Autodesk Inventor part; units mm, degrees
ref_plane "YZ Plane" through (0, 0, 0) normal (1, 0, 0) x (0, 1, 0)
ref_plane "XZ Plane" through (0, 0, 0) normal (0, 1, 0) x (-1, 0, 0)
ref_plane "XY Plane" through (0, 0, 0) normal (0, 0, 1) x (1, 0, 0)
sketch "Sketch1" plane through (0, 0, 0) normal (0, 0, 1) x (1, 0, 0)
  circle A0 centre (0, 0) radius 18.5
  dimension "d0" = 37
extrude "Extrusion1" add sketch "Sketch1" along normal blind 85
sketch "Sketch2" plane through (0, 0, 85) normal (0, 0, 1) x (1, 0, 0)
  circle A0 centre (0, -7) radius 3
  point P0 (0, 0)
  dimension "d3" = 6
  dimension "d4" = 7
extrude "Extrusion2" add sketch "Sketch2" along normal blind 21
sketch "Sketch3" plane through (0, 0, 85) normal (0, 0, 1) x (1, 0, 0)
  circle A0 centre (0, -7) radius 3
  circle A1 centre (0, -7) radius 6
  point P0 (0, 0)
  dimension "d7" = 12
extrude "Extrusion3" add sketch "Sketch3" along normal blind 6
sketch "Sketch4" plane through (0, -7, 106) normal (0, 0, 1) x (1, 0, 0)
  circle A0 centre (0, 0) radius 3
  line L0 (-1.8, 2.4) -> (1.8, 2.4)
  point P0 (0, 7)
  dimension "d10" = 2.4
extrude "Extrusion4" cut sketch "Sketch4" against normal blind 12 contours L0 A0 picked at (0, 2.6)
sketch "Sketch5" plane through (0, 0, 85) normal (0, 0, 1) x (1, 0, 0)
  circle A0 centre (15.5, 0) radius 1.5
  circle A1 centre (7.75, 13.4234) radius 1.5
  circle A2 centre (-7.75, 13.4234) radius 1.5
  circle A3 centre (-15.5, 0) radius 1.5
  circle A4 centre (-7.75, -13.4234) radius 1.5
  circle A5 centre (7.75, -13.4234) radius 1.5
  point P0 (0, 0)
  dimension "d13" = 3
  dimension "d14" = 15.5
  dimension "d17" = 360
extrude "Extrusion5" cut sketch "Sketch5" against normal blind 12
properties material "Steel, Carbon"
Build history of the part. All positions in model axes, mm. A direction names the side the tool comes from. Round coordinates to 2 decimals unless told otherwise and drop trailing zeros. Write each loop counter-clockwise with the first axis right and the second up, starting at its lowest first coordinate (ties: lowest second). Pieces come first, ordered by that corner, then holes. Notation, with made-up numbers: M 54,83.5 L 104,83.5 A31 ccw 104,118.5 Z; hole C 35.5,73 d4. An arc over 180 degrees is marked long. Answer in a Markdown table with one row per item.
1. Saw through at D-D (z = 17.5). List the corners of the cut face in (x, y).
Geometry check:
| item | result |
|---|---|
| outline | C 0,0 d37 |
2. Saw through at B-B (z = 74). List the corners of the cut face in (x, y), and give its area (3 significant figures).
Geometry check:
| item | result |
|---|---|
| outline | C 0,0 d37; hole C -15.5,0 d3; hole C -7.75,-13.42 d3; hole C -7.75,13.42 d3; hole C 7.75,-13.42 d3; hole C 7.75,13.42 d3; hole C 15.5,0 d3 |
| area | 1,030 mm2 |
3. Which spindle directions (+Z, -Z, +X, -X, +Y, -Y) get a long thin tool onto all of the face, cutting with end or side? Do faces 1 (the face through (-8.856, -12.41, 79.084)), 2 (the face through (0, 0, 0)). Say none if no direction does.
Geometry check:
| item | result |
|---|---|
| face 1 | +Z |
| face 2 | -Z, +X, -X, +Y, -Y |
4. Saw through at A-A (x = 15.5). List the corners of the cut face in (y, z), and give its area (3 significant figures).
Geometry check:
| item | result |
|---|---|
| outline | M -10.1,0 L 10.1,0 L 10.1,85 L 1.5,85 L 1.5,73 L -1.5,73 L -1.5,85 L -10.1,85 Z |
| area | 1,680 mm2 |
5. Flat gauge pins, fed straight in: P1, Ø1.8, axis at x = 7.75, y = -13.42, coming from the -Z side; P2, Ø1.5, axis at x = -15.5, y = 0.5, coming from the +Z side; P3, Ø1.8, axis at x = 0, z = 98.5, coming from the +Y side; P4, Ø2, axis at x = -13.5, y = -4.5, coming from the +Z side. Where does each tip first touch, or does it go through?
Geometry check:
| item | result |
|---|---|
| P1 | z = 0 |
| P2 | z = 73 |
| P3 | y = -4.6 |
| P4 | z = 85 |
6. Probe L1, parallel to Y at x = 7.75, z = 77; L2, parallel to X at y = -7, z = 92.5; L3, parallel to Z at x = -6.5, y = -4. List the from-to ranges inside material, lowest first. Write a range as [from, to].
Geometry check:
| item | result |
|---|---|
| L1 | [-16.8, -14.92], [-11.92, 11.92], [14.92, 16.8] |
| L2 | [-3, 3] |
| L3 | [0, 85] |
7. Saw through at C-C (y = -7). List the corners of the cut face in (x, z), and give its area (3 significant figures).
Geometry check:
| item | result |
|---|---|
| outline | M -17.12,0 L 17.12,0 L 17.12,85 L 6,85 L 6,91 L 3,91 L 3,106 L -3,106 L -3,91 L -6,91 L -6,85 L -17.12,85 Z |
| area | 3,070 mm2 |
8. Mould opens along Y. For faces 3 (the face through (0, 0, 85)), 4 (the face through (0, -4.6, 100)), 5 (the face through (-8, -13, 73)) say: +Y half, -Y half, draft (parallel to the pull), parting line (faces both ways), or undercut.
Geometry check:
| item | result |
|---|---|
| face 3 | draft |
| face 4 | +Y half |
| face 5 | undercut |
